Autodesk Inventor part; units mm, degrees
ref_plane "Cross Section Plane" through (5.8114, -5.4363, 0) normal (0.6831, 0.7303, 0) x (0, 0, 1)
ref_plane "Work Plane2" through (0, 0, 0) normal (-1, 0, 0) x (0, 0, 1)
ref_plane "Work Plane3" through (0.2486, 112.4632, 0) normal (0.155, -0.9879, 0) x (0, 0, 1)
sketch "Sketch Path" plane through (0, 0, 0) normal (0, 0, 1) x (1, 0, 0)
  arc A0 (-7.7801, -1.672) -> (5.8114, -5.4363) centre (0, 0) ccw
  arc A1 (28.9379, 126.2523) -> (-30.8718, 105.775) centre (0.2486, 112.4632) ccw
  arc A2 (58.2507, 50.621) -> (59.9518, 61.7255) centre (50.9864, 57.4164) ccw
  line L0 (58.2507, 50.621) -> (5.8114, -5.4363)
  line L1 (-7.7801, -1.672) -> (-30.8718, 105.775)
  line L2 (28.9379, 126.2523) -> (59.9518, 61.7255)
ref_plane "Cross Section Plane" through (5.8114, -5.4363, 0) normal (0.6831, 0.7303, 0) x (0, 0, 1)
ref_plane "Work Plane2" through (0, 0, 0) normal (-1, 0, 0) x (0, 0, 1)
ref_plane "Work Plane3" through (0.2486, 112.4632, 0) normal (0.155, -0.9879, 0) x (0, 0, 1)
ref_plane "Work Plane4" through (50.9864, 57.4164, 0) normal (-0.4137, 0.9104, 0) x (0, 0, 1)
sketch "Cross Section" plane through (5.8114, -5.4363, 0) normal (0.6831, 0.7303, 0) x (0, 0, 1)
  line L0 (-3, 0.3) -> (3, 0.3)
  line L1 (3, 0.3) -> (3, -0.3)
  line L2 (3, -0.3) -> (-3, -0.3)
  line L3 (-3, -0.3) -> (-3, 0.3)
  line L4 (-3, 0) -> (3, 0) construction
  point P0 (0, 0)
  point P1 (0, 0)
  dimension "d0" = 6
  dimension "d4" = 0.3
  dimension "d5" = 0.3
sweep "Belt" add profiles "Cross Section" path "Sketch Path"
equation "\"d0\" = da_B"
equation "\"d4\" = da_a"
equation "\"d5\" = da_a2"
equation "\"da_B\" = 6"
equation "\"da_pb\" = 2.5"
equation "\"da_a\" = 0.3"
equation "\"da_S\" = 1.5"
equation "\"da_Beta\" = 20deg"
equation "\"da_Ht\" = 0.7"
equation "\"da_H\" = 1.3"
equation "\"da_a2\" = 0.3"
properties part number "Synchronous Belt" material "Rubber"
Can you work these out from the model? Positions are in its coordinate system, mm. A direction names the side the tool comes from. Give positions to 0.01 mm unless a question says otherwise; leave off trailing zeros. Order: outer loops, then holes, each group sorted by start corner. A loop starts at its lowest first (then second) coordinate and runs counter-clockwise, first axis right, second up. Notation, with made-up numbers: M 59,-14.5 L 64,-14.5 A19 ccw 64,7.5 Z; hole C 33.25,22.5 d6. An arc over 180 degrees is marked long. Write item = value, one per line. Start each with the question number.
Q1. For faces 1 (the cylindrical face through (-2.156, -7.348, 0.042)), 2 (the cylindrical face through (-2.08, -7.99, -0.04)), which set-ups out of +Z, -Z, +X, -X, +Y, -Y let a thin tool reach every point of the face, with its end or its side?
Q2. We'd pull the mould along X, two halves only. Please class faces 3 (the cylindrical face through (-9.356, 142.496, 0.042)), 4 (the flat face through (32.62, 22.78, 0.04)), 5 (the cylindrical face through (-10.775, 142.644, -0.042)): pulls with the +X half, pulls with the -X half, needs draft (parallel to the pull), parting line crosses it, or undercut.
Q3. Suppose I cut it at C-C (y = 83). Write out the boundary of the cut face in (x, z).
Q4. Suppose I cut it at B-B (x = -13.5). Write out the boundary of the cut face in (y, z).
Q5. Suppose I cut it at A-A (z = 1.55). Write out the boundary of the cut face in (x, y), plus the area to 3 significant figures.
Q6. I need wall thicknesses on probe 1 along Y at (x, z) = (0, -1.15); probe 2 along Y at (x, z) = (46, -1.5); probe 3 along X at (y, z) = (102.5, -1.35). Which ranges of each line are inside material? Lowest first, please. Write a range as [from, to].
Q7. Will these pins go through, and if not, where does the flat tip stop? pin 1 Ø1 at (x, z) = (-1, 1) entering from +Y; pin 2 Ø2 at (y, z) = (75.5, -1.5) entering from +X; pin 3 Ø2 at (y, z) = (53.5, -1.5) entering from -X.
Check result:
q1.face_1 = +Z, -Z
q1.face_2 = +Z, -Z, -Y
q2.face_3 = undercut
q2.face_4 = pulls with the +X half
q2.face_5 = parting line crosses it
q3.outline = M -26.28,-3 L -25.67,-3 L -25.67,3 L -26.28,3 Z; M 49.39,-3 L 50.06,-3 L 50.06,3 L 49.39,3 Z
q4.outline = M 23.52,-3 L 26.37,-3 L 26.37,3 L 23.52,3 Z; M 140.84,-3 L 141.5,-3 L 141.5,3 L 140.84,3 Z
q5.outline = M -31.17,105.71 L -8.07,-1.74 A8.26 ccw 6.03,-5.64 L 58.47,50.42 A10.25 ccw 60.22,61.86 L 29.21,126.38 A32.13 ccw Z; hole M -30.58,105.84 L -7.49,-1.61 A7.66 ccw 5.59,-5.23 L 58.03,50.83 A9.65 ccw 59.68,61.6 L 28.67,126.12 A31.53 ccw Z
q5.area = 228 mm2
q6.probe_1 = [-8.26, -7.66], [143.99, 144.59]
q6.probe_2 = [37.09, 37.96], [90.06, 91.45]
q6.probe_3 = [-30.47, -29.86], [40.02, 40.69]
q7.pin_1 = 144.59
q7.pin_2 = 54.14
q7.pin_3 = -20.16
